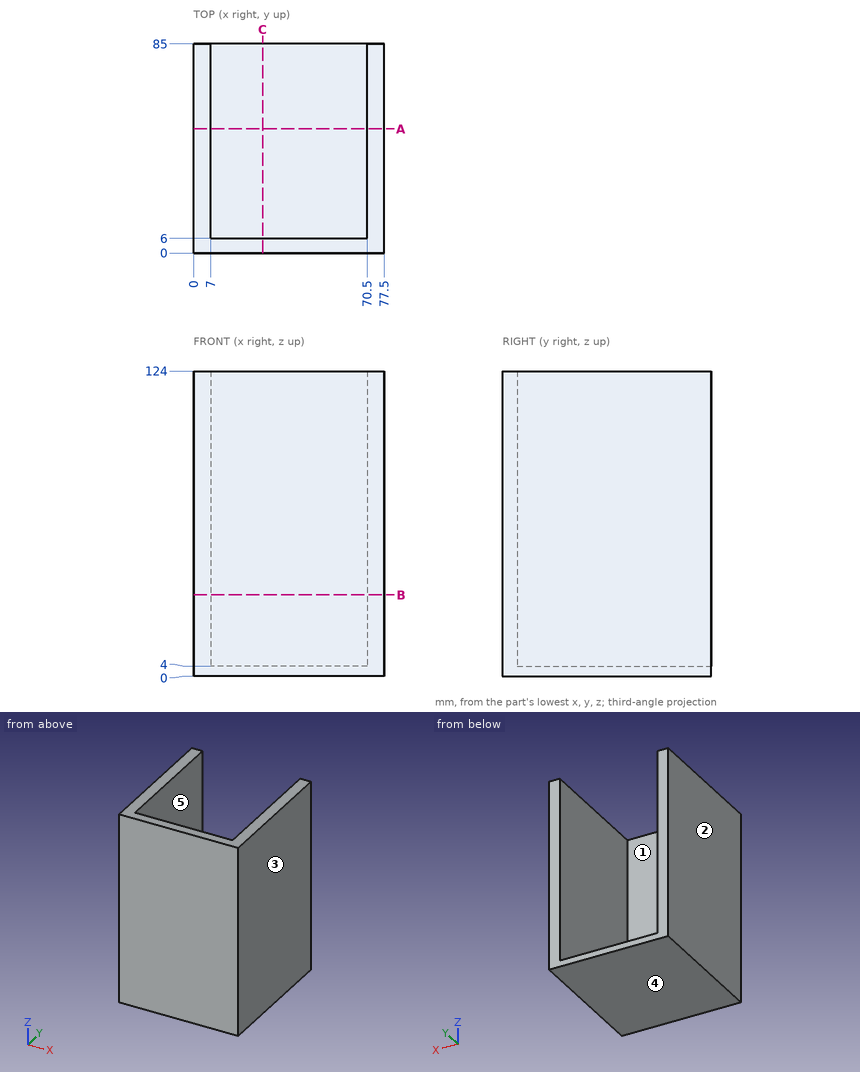
Part print with two shaded views. Sizes in mm from the minimum x, y, z corner. A direction names the side the tool comes from. Round coordinates to 2 decimals unless told otherwise and drop trailing zeros. Order: outer loops, then holes, each group sorted by start corner. A loop starts at its lowest first (then second) coordinate and runs counter-clockwise, first axis right, second up.
(1) 3-axis set-ups, long thin cutter, end or side, ignore diameter. For the marked faces 1 and 2: which of +Z, -Z, +X, -X, +Y, -Y reach the whole face in a straight line?
(2) Pull direction X, two halves, no side cores. Call the marked faces 3, 4 and 5: released by +X, released by -X, zero draft, split by the parting line, or undercut.
(3) Drill centre lines: line 1 (X direction, y = 79, z = 73); line 2 (Y direction, x = 8, z = 104); line 3 (Z direction, x = 15.5, y = 69.5). Where is each one in solid material? Low to high.
(4) Band-saw the part on C-C (x = 28). List the corners of the cut face in (y, z), then the cut area to 3 significant figures.
(5) Pin check, flat tips, straight feed: pin 1 (6 mm diameter, centred on x = 16, y = 17, fed in from +Z); pin 2 (2 mm diameter, centred on x = 13.5, y = 64.5, fed in from -Z); pin 3 (5 mm diameter, centred on x = 32.5, z = 97, fed in from +Y). Stop position of each tip, or through.
(6) Band-saw the part on A-A (y = 50.5). List the corners of the cut face in (x, z).
(7) Band-saw the part on B-B (z = 33). List the corners of the cut face in (x, y).
Verdict:
1. face 1: +Z, +Y
1. face 2: +Z, -Z, -X, +Y, -Y
2. face 3: released by +X
2. face 4: zero draft
2. face 5: undercut
3. line 1: x = 0 to 7, 70.5 to 77.5
3. line 2: y = 0 to 6
3. line 3: z = 0 to 4
4. outline: (0, 0) - (85, 0) - (85, 4) - (6, 4) - (6, 124) - (0, 124) - close
4. area: 1,060 mm2
5. pin 1: stops at z = 4
5. pin 2: stops at z = 0
5. pin 3: stops at y = 6
6. outline: (0, 0) - (77.5, 0) - (77.5, 124) - (70.5, 124) - (70.5, 4) - (7, 4) - (7, 124) - (0, 124) - close
7. outline: (0, 0) - (77.5, 0) - (77.5, 85) - (70.5, 85) - (70.5, 6) - (7, 6) - (7, 85) - (0, 85) - close
